```python
from build123d import *

# Parameters (mm, degrees)
SKETCH2_R           = 1.65
SKETCH2_R_2         = 11
SKETCH2_R_3         = 1.5
SKETCH2_R_4         = 1
BOSS_EXTRUDE1_DEPTH = 4


with BuildPart() as part:
    # Sketch2 → Boss-Extrude1 (new body)
    with BuildSketch(Plane.XY):
        with BuildLine():
            Line((-140, 175), (-118.205067931, 175))
            ThreePointArc((-118.205067931, 175), (-113.316837275, 173.723829494), (-109.676249776, 170.221040209))
            add(Edge.make_bspline(
                [(-109.676249776, 170.221040209), (-107.076087276, 165.973550773), (-102.14217925, 162.295269988), (-97.095196953, 162)],
                knots=[0.25103648, 0.25103648, 0.25103648, 0.25103648, 1, 1, 1, 1], degree=3))
            Line((-97.095196953, 162), (97.095196953, 162))
            add(Edge.make_bspline(
                [(109.676249776, 170.221040209), (107.076087276, 165.973550773), (102.14217925, 162.295269988), (97.095196953, 162)],
                knots=[0.25103648, 0.25103648, 0.25103648, 0.25103648, 1, 1, 1, 1], degree=3))
            ThreePointArc((109.676249776, 170.221040209), (113.316837275, 173.723829494), (118.205067931, 175))
            Line((118.205067931, 175), (140, 175))
            ThreePointArc((140, 175), (143.535533906, 173.535533906), (145, 170))
            Line((145, 170), (145, 57))
            ThreePointArc((145, 57), (144.414213562, 55.585786438), (143, 55))
            Line((143, 55), (132, 55))
            ThreePointArc((132, 55), (130.585786438, 54.414213562), (130, 53))
            Line((130, 53), (130, -3))
            ThreePointArc((130, -3), (130.585786438, -4.414213562), (132, -5))
            Line((132, -5), (143, -5))
            ThreePointArc((143, -5), (144.414213562, -5.585786438), (145, -7))
            Line((145, -7), (145, -120))
            ThreePointArc((145, -120), (143.535533906, -123.535533906), (140, -125))
            Line((140, -125), (118.205067931, -125))
            ThreePointArc((118.205067931, -125), (113.316837275, -123.723829494), (109.676249776, -120.221040209))
            add(Edge.make_bspline(
                [(109.676249776, -120.221040209), (107.076087276, -115.973550773), (102.14217925, -112.295269988), (97.095196953, -112)],
                knots=[0.25103648, 0.25103648, 0.25103648, 0.25103648, 1, 1, 1, 1], degree=3))
            Line((97.095196953, -112), (-97.095196953, -112))
            add(Edge.make_bspline(
                [(-109.676249776, -120.221040209), (-107.076087276, -115.973550773), (-102.14217925, -112.295269988), (-97.095196953, -112)],
                knots=[0.25103648, 0.25103648, 0.25103648, 0.25103648, 1, 1, 1, 1], degree=3))
            ThreePointArc((-109.676249776, -120.221040209), (-113.316837275, -123.723829494), (-118.205067931, -125))
            Line((-118.205067931, -125), (-140, -125))
            ThreePointArc((-140, -125), (-143.535533906, -123.535533906), (-145, -120))
            Line((-145, -120), (-145, -7))
            ThreePointArc((-145, -7), (-144.414213562, -5.585786438), (-143, -5))
            Line((-143, -5), (-132, -5))
            ThreePointArc((-132, -5), (-130.585786438, -4.414213562), (-130, -3))
            Line((-130, -3), (-130, 53))
            ThreePointArc((-130, 53), (-130.585786438, 54.414213562), (-132, 55))
            Line((-132, 55), (-143, 55))
            ThreePointArc((-143, 55), (-144.414213562, 55.585786438), (-145, 57))
            Line((-145, 57), (-145, 170))
            ThreePointArc((-145, 170), (-143.535533906, 173.535533906), (-140, 175))
        make_face()
        with Locations((-132.473303105, 168.56037538)):
            Circle(SKETCH2_R, mode=Mode.SUBTRACT)
        with Locations((-132.473303105, 139.890769728)):
            Circle(SKETCH2_R, mode=Mode.SUBTRACT)
        with Locations((132.473303105, 168.56037538)):
            Circle(SKETCH2_R, mode=Mode.SUBTRACT)
        with Locations((132.473303105, 139.890769728)):
            Circle(SKETCH2_R, mode=Mode.SUBTRACT)
        with Locations((132.473303105, 154.225572554)):
            Circle(SKETCH2_R_2, mode=Mode.SUBTRACT)
        with Locations((-132.473303105, 154.225572554)):
            Circle(SKETCH2_R_2, mode=Mode.SUBTRACT)
        with Locations((121.59774802, -0.5)):
            Circle(SKETCH2_R, mode=Mode.SUBTRACT)
        with Locations((121.59774802, 50.5)):
            Circle(SKETCH2_R, mode=Mode.SUBTRACT)
        with Locations((-121.59774802, -0.5)):
            Circle(SKETCH2_R, mode=Mode.SUBTRACT)
        with Locations((-121.59774802, 50.5)):
            Circle(SKETCH2_R, mode=Mode.SUBTRACT)
        with Locations((-29, 10)):
            Circle(SKETCH2_R_3, mode=Mode.SUBTRACT)
        with Locations((-29, 40)):
            Circle(SKETCH2_R_3, mode=Mode.SUBTRACT)
        with Locations((-53, 40)):
            Circle(SKETCH2_R_3, mode=Mode.SUBTRACT)
        with Locations((-53, 10)):
            Circle(SKETCH2_R_3, mode=Mode.SUBTRACT)
        with Locations((53, 10)):
            Circle(SKETCH2_R_3, mode=Mode.SUBTRACT)
        with Locations((29, 10)):
            Circle(SKETCH2_R_3, mode=Mode.SUBTRACT)
        with Locations((29, 40)):
            Circle(SKETCH2_R_3, mode=Mode.SUBTRACT)
        with Locations((53, 40)):
            Circle(SKETCH2_R_3, mode=Mode.SUBTRACT)
        with Locations((132.473303105, -118.56037538)):
            Circle(SKETCH2_R, mode=Mode.SUBTRACT)
        with Locations((132.473303105, -89.890769728)):
            Circle(SKETCH2_R, mode=Mode.SUBTRACT)
        with Locations((132.473303105, -104.225572554)):
            Circle(SKETCH2_R_2, mode=Mode.SUBTRACT)
        with Locations((-132.473303105, -104.225572554)):
            Circle(SKETCH2_R_2, mode=Mode.SUBTRACT)
        with Locations((-132.473303105, -89.890769728)):
            Circle(SKETCH2_R, mode=Mode.SUBTRACT)
        with Locations((-132.473303105, -118.56037538)):
            Circle(SKETCH2_R, mode=Mode.SUBTRACT)
        with Locations((130, 75)):
            Circle(SKETCH2_R_3, mode=Mode.SUBTRACT)
        with Locations((41.5, 95.575)):
            Circle(SKETCH2_R_4, mode=Mode.SUBTRACT)
        with Locations((41.5, 80.575)):
            Circle(SKETCH2_R_4, mode=Mode.SUBTRACT)
        with Locations((-20, 80.575)):
            Circle(SKETCH2_R_4, mode=Mode.SUBTRACT)
        with Locations((-20, 95.575)):
            Circle(SKETCH2_R_4, mode=Mode.SUBTRACT)
        with Locations((-20, -45.575)):
            Circle(SKETCH2_R_4, mode=Mode.SUBTRACT)
        with Locations((-20, -30.575)):
            Circle(SKETCH2_R_4, mode=Mode.SUBTRACT)
        with Locations((41.5, -30.575)):
            Circle(SKETCH2_R_4, mode=Mode.SUBTRACT)
        with Locations((41.5, -45.575)):
            Circle(SKETCH2_R_4, mode=Mode.SUBTRACT)
        with Locations((130, -25)):
            Circle(SKETCH2_R_3, mode=Mode.SUBTRACT)
        with Locations((-130, 75)):
            Circle(SKETCH2_R_3, mode=Mode.SUBTRACT)
        with Locations((-130, -25)):
            Circle(SKETCH2_R_3, mode=Mode.SUBTRACT)
        with BuildLine():
            Line((-66, 62.171403079), (-111.59774802, 62.171403079))
            ThreePointArc((-111.59774802, 62.171403079), (-114.426175145, 60.999830204), (-115.59774802, 58.171403079))
            Line((-115.59774802, 58.171403079), (-115.59774802, -8.171403079))
            ThreePointArc((-115.59774802, -8.171403079), (-114.426175145, -10.999830204), (-111.59774802, -12.171403079))
            Line((-111.59774802, -12.171403079), (-66, -12.171403079))
            ThreePointArc((-66, -12.171403079), (-63.171572875, -10.999830204), (-62, -8.171403079))
            Line((-62, -8.171403079), (-62, 58.171403079))
            ThreePointArc((-62, 58.171403079), (-63.171572875, 60.999830204), (-66, 62.171403079))
        make_face(mode=Mode.SUBTRACT)
        with BuildLine():
            Line((66, 62.171403079), (111.59774802, 62.171403079))
            ThreePointArc((111.59774802, 62.171403079), (114.426175145, 60.999830204), (115.59774802, 58.171403079))
            Line((115.59774802, 58.171403079), (115.59774802, -8.171403079))
            ThreePointArc((115.59774802, -8.171403079), (114.426175145, -10.999830204), (111.59774802, -12.171403079))
            Line((111.59774802, -12.171403079), (66, -12.171403079))
            ThreePointArc((66, -12.171403079), (63.171572875, -10.999830204), (62, -8.171403079))
            Line((62, -8.171403079), (62, 58.171403079))
            ThreePointArc((62, 58.171403079), (63.171572875, 60.999830204), (66, 62.171403079))
        make_face(mode=Mode.SUBTRACT)
    extrude(amount=BOSS_EXTRUDE1_DEPTH)


solid = part.part
```
Part model, mm, in its own coordinate system. Round coordinates to 2 decimals unless told otherwise and drop trailing zeros. Order: outer loops, then holes, each group sorted by start corner. A loop starts at its lowest first (then second) coordinate and runs counter-clockwise, first axis right, second up. Notation, with made-up numbers: M 71.5,-3.75 L 102.5,-3.75 A32 cw 102.5,23.25 Z; hole C 13.25,3.5 d7. An arc over 180 degrees is marked long. Put each result on its own line as item: value. Start each with the question number.
1. Slice it at B-B on x = 89. List the corners of the cut face in (y, z), then the cut area to 3 significant figures.
2. Slice it at C-C on x = -41. List the corners of the cut face in (y, z), then the cut area to 3 significant figures.
3. Two-plate mould, pull along X, no slides. Class faces 1 (the face through (2, 27, 0)), 2 (the face through (121.484, 154.709, 1.972)): +X half, -X half, draft (parallel to the pull), parting line (faces both ways), or undercut.
4. Drop flat-ended pins along their axis: pin 1 (1.2 mm diameter, centred on x = -41.5, z = 2.5, fed in from +Y); pin 2 (2 mm diameter, centred on x = -37.5, z = 2.5, fed in from -Y); pin 3 (1.2 mm diameter, centred on y = 27.5, z = 2.5, fed in from -X). Give the stop position or say it passes through.
5. Slice it at A-A on y = 15.5. List the corners of the cut face in (x, z).
6. Slice it at D-D on z = 0.85. State how many separate pieces and enclosed holes the cut face has, then the cut area to 3 significant figures.
7. Drill centre lines: probe 1 along X at (y, z) = (48, 0.2); probe 2 along Y at (x, z) = (53, 2); probe 3 along X at (y, z) = (75, 2.5). Where is each one in solid material? Low to high. Write a range as [from, to].
Findings:
1. outline: M -112,0 L -12.17,0 L -12.17,4 L -112,4 Z; M 62.17,0 L 162,0 L 162,4 L 62.17,4 Z
1. area: 799 mm2
2. outline: M -112,0 L 162,0 L 162,4 L -112,4 Z
2. area: 1,100 mm2
3. face 1: draft
3. face 2: undercut
4. pin 1: y = 162
4. pin 2: y = -112
4. pin 3: x = -130
5. outline: M -130,0 L -115.6,0 L -115.6,4 L -130,4 Z; M -62,0 L 62,0 L 62,4 L -62,4 Z; M 115.6,0 L 130,0 L 130,4 L 115.6,4 Z
6. separate pieces: 1
6. enclosed holes: 38
6. area: 69,900 mm2
7. probe 1: [-130, -115.6], [-62, 62], [115.6, 130]
7. probe 2: [-112, 8.5], [11.5, 38.5], [41.5, 162]
7. probe 3: [-145, -131.5], [-128.5, 128.5], [131.5, 145]
